Autodesk Inventor part; units mm, degrees
ref_plane "YZ Plane" through (0, 0, 0) normal (1, 0, 0) x (0, 1, 0)
ref_plane "XZ Plane" through (0, 0, 0) normal (0, 1, 0) x (-1, 0, 0)
ref_plane "XY Plane" through (0, 0, 0) normal (0, 0, 1) x (1, 0, 0)
sketch "Sketch1" plane through (0, 0, 0) normal (0, 0, 1) x (1, 0, 0)
  line L0 (0, 0) -> (97.5, 0)
  line L1 (97.5, 0) -> (97.5, 9)
  line L2 (97.5, 9) -> (0, 9)
  line L3 (0, 9) -> (0, 0)
  dimension "d2" = 97.5
  dimension "d3" = 9
extrude "Extrusion1" add sketch "Sketch1" along normal blind 6
sketch "Sketch2" plane through (0, 0, 6) normal (0, 0, 1) x (1, 0, 0)
  line L0 (0, 0) -> (97.5, 0)
  line L1 (97.5, 0) -> (97.5, 9)
  line L2 (0, 9) -> (0, 0)
  line L3 (2, 0) -> (32.5, 0)
  line L4 (32.5, 0) -> (32.5, 9)
  line L5 (32.5, 9) -> (2, 9)
  line L6 (2, 9) -> (2, 0)
  line L7 (33.5, 9) -> (64, 9)
  line L8 (64, 9) -> (64, 0)
  line L9 (64, 0) -> (33.5, 0)
  line L10 (33.5, 0) -> (33.5, 9)
  line L11 (65, 0) -> (95.5, 0)
  line L12 (95.5, 0) -> (95.5, 9)
  line L13 (95.5, 9) -> (65, 9)
  line L14 (65, 9) -> (65, 0)
  line L15 (97.5, 9) -> (0, 9)
  dimension "d5" = 30.5
  dimension "d6" = 2
  dimension "d7" = 2
  dimension "d8" = 30.5
  dimension "d9" = 30.5
  dimension "d10" = 1
extrude "Extrusion2" cut sketch "Sketch2" against normal blind 3 contours L6 L5 L4 L0 | L10 L7 L8 L0 | L14 L13 L12 L0
sketch "Sketch7" plane through (0, 0, 0) normal (0, 0, -1) x (-1, 0, 0)
  line L0 (0, 0) -> (-97.5, 0)
  line L1 (0, 9) -> (0, 0)
  line L2 (-97.5, 9) -> (0, 9)
  line L3 (-97.5, 0) -> (-97.5, 9)
  line L4 (-82.25, 7) -> (-15.25, 7)
  line L5 (-15.25, 7) -> (-15.25, 2)
  line L6 (-15.25, 2) -> (-82.25, 2)
  line L7 (-82.25, 2) -> (-82.25, 7)
  line L8 (-82.25, 7) -> (-15.25, 2) construction
  line L9 (-15.25, 7) -> (-82.25, 2) construction
  line L10 (-48.75, 9) -> (-48.75, 0) construction
  line L11 (-97.5, 4.5) -> (0, 4.5) construction
  point P0 (-48.75, 4.5)
  point P1 (-48.75, 4.5)
  point P2 (-48.75, 4.5)
  dimension "d31" = 67
  dimension "d32" = 5
extrude "Extrusion7" cut sketch "Sketch7" against normal blind 10 contours L4 L5 L6 L7
fillet "Fillet1" radius 2 2 edges at (97.5, 4.5, 0) (0, 4.5, 0)
properties part number "base_corner" material "ABS Plastic"
Can you work these out from the model? Positions are in its coordinate system, mm. A direction names the side the tool comes from. Coordinates: 2 decimals unless noted, no trailing zeros. Write each loop counter-clockwise with the first axis right and the second up, starting at its lowest first coordinate (ties: lowest second). Pieces come first, ordered by that corner, then holes. Notation, with made-up numbers: M 74,83 L 78,83 A17 ccw 78,90 Z; hole C 34,9.5 d3. An arc over 180 degrees is marked long. Use one line per item in the form item = value.
Q1. For P1, Ø0.6, axis at x = 46.5, y = 8, coming from the +Z side, with a flat end and sliding along its axis, tell me the tip position at first contact or that it passes through.
Model answer:
P1 = 3
Q2. For faces 1 (the flat face through (49, 7, 2)), 2 (the flat face through (97.5, 4, 4)), 3 (the flat face through (65, 8, 5)), which set-ups out of +Z, -Z, +X, -X, +Y, -Y let a thin tool reach every point of the face, with its end or its side?
Model answer:
face_1 = +Z, -Z
face_2 = +Z, -Z, +X, +Y, -Y
face_3 = +Z, +Y, -Y
Q3. If we section it at C-C (z = 4.15): Write out the boundary of the cut face in (x, y), then the cut area to 3 significant figures.
Model answer:
outline = M 0,0 L 2,0 L 2,9 L 0,9 Z; M 32.5,0 L 33.5,0 L 33.5,2 L 32.5,2 Z; M 32.5,7 L 33.5,7 L 33.5,9 L 32.5,9 Z; M 64,0 L 65,0 L 65,2 L 64,2 Z; M 64,7 L 65,7 L 65,9 L 64,9 Z; M 95.5,0 L 97.5,0 L 97.5,9 L 95.5,9 Z
area = 44.0 mm^2
Q4. If we section it at A-A (y = 4): Write out the boundary of the cut face in (x, z), then the cut area to 3 significant figures.
Model answer:
outline = M 0,2 A2 ccw 2,0 L 15.25,0 L 15.25,3 L 2,3 L 2,6 L 0,6 Z; M 82.25,0 L 95.5,0 A2 ccw 97.5,2 L 97.5,6 L 95.5,6 L 95.5,3 L 82.25,3 Z
area = 102 mm^2
Q5. We'd pull the mould along Y, two halves only. Please class faces 4 (the flat face through (48, 0, 2)), 5 (the flat face through (48.1, 1.6, 0)), 6 (the flat face through (82.25, 4, 1)): +Y half, -Y half, draft (parallel to the pull), parting line (faces both ways), or undercut.
Model answer:
face_4 = -Y half
face_5 = draft
face_6 = undercut
Q6. If we section it at B-B (x = 20): Write out the boundary of the cut face in (y, z), then the cut area to 3 significant figures.
Model answer:
outline = M 0,0 L 2,0 L 2,3 L 0,3 Z; M 7,0 L 9,0 L 9,3 L 7,3 Z
area = 12.0 mm^2
Q7. I need wall thicknesses on line 1 along X through (y, z) = (8.5, 5.35); line 2 along X through (y, z) = (4.75, 4.65); line 3 along Y through (x, z) = (26, 1.4). Which ranges of each line are inside material? Lowest first, please. Write a range as from..to.
Model answer:
line_1 = 0..2, 32.5..33.5, 64..65, 95.5..97.5
line_2 = 0..2, 95.5..97.5
line_3 = 0..2, 7..9
